Geometry: final body of the model. Coordinates: model frame, mm. A direction names the side the tool comes from. Give positions to 0.01 mm unless a question says otherwise; leave off trailing zeros. Write each loop counter-clockwise with the first axis right and the second up, starting at its lowest first coordinate (ties: lowest second). Pieces come first, ordered by that corner, then holes. Notation, with made-up numbers: (-6.5, 38.25) -> (27.5, 38.25) arc R28 ccw to (27.5, 65.25) -> close; hole circle Ø2 at (9.5, 31). An arc over 180 degrees is marked (long way). Answer in a Markdown table with one row per item. Add a question column.
Item 1: Material intervals for probe 1 along Z at (x, y) = (0, 4); probe 2 along Y at (x, z) = (12, -5.25); probe 3 along Z at (x, y) = (0, 48), sorted ascending. Write a range as from..to.
Item 2: Section query B-B on z = 0. Output: boundary loops of the cut face in (x, y), plus the area to 3 significant figures.
Item 3: Section query C-C on y = 80.5. Output: boundary loops of the cut face in (x, z), plus the area to 3 significant figures.
Item 4: Draft query along X for faces 4 (the cylindrical face through (14.07, 11.89, 4.43)), 5 (the flat face through (0, 77.8, 0)), 6 (the flat face through (-1, 12.9, -12)). Return one class per face: +X half, -X half, draft (parallel to the pull), parting line (faces both ways), or undercut.
Item 5: First-contact query: P1, Ø8, axis at x = -8.5, y = 20, coming from the +Z side; P2, Ø1.5, axis at y = 74.5, z = -6.5, coming from the +X side; P3, Ø8, axis at x = 7, y = 16.5, coming from the -Z side. Flat tips, straight axial feed; report the tip coordinate or a pass-through.
Item 6: Section query A-A on x = 0. Output: boundary loops of the cut face in (y, z).
Item 7: Section query D-D on y = 58. Output: boundary loops of the cut face in (x, z), plus the area to 3 significant figures.
Item 8: Access query for faces 1 (the cylindrical face through (11.207, 43.466, 3.529)), 2 (the flat face through (0, 10, 0)), 3 (the cylindrical face through (0, 83, -2)). Directions: +Z, -Z, +X, -X, +Y, -Y. A direction counts if a zero-diameter tool reaches every point of the face in a straight line with its end or side. Return the directions, or none.
Autodesk Fusion 360 part; units mm, degrees
sketch "Sketch1" plane through (0, 0, 0) normal (0, 1, 0) x (1, 0, 0)
  circle A0 centre (0, 0) radius 11.75
  dimension "d1" = 23.5
extrude "Extrude1" add sketch "Sketch1" along normal blind 87.8
sketch "Sketch2" plane through (0, 0, 0) normal (0, -1, 0) x (1, 0, 0)
  circle A0 centre (0, 0) radius 11.75
  circle A1 centre (0, 0) radius 2
  dimension "d4" = 4
extrude "Extrude2" cut sketch "Sketch2" against normal blind 10 contours A1
sketch "Sketch3" plane through (0, 87.8, 0) normal (0, 1, 0) x (-1, 0, 0)
  circle A0 centre (0, 0) radius 11.75
  circle A1 centre (0, 0) radius 2
  dimension "d7" = 4
extrude "Extrude3" cut sketch "Sketch3" against normal blind 10 contours A1
sketch "Sketch4" plane through (0, 0, 0) normal (0, -1, 0) x (1, 0, 0)
  circle A0 centre (0, 0) radius 2
  circle A1 centre (0, 0) radius 11.75
  circle A2 centre (0, 0) radius 14.75
  dimension "d10" = 3
extrude "Extrude4" add sketch "Sketch4" against normal blind 2 from surface at -10.9 contours A2
extrude "Extrude5" add sketch "Sketch4" along normal blind 2 from surface at -76.9 contours A2
Findings below:
| question | item | result |
|---|---|---|
| 1 | probe 1 | z = -11.75..-2, 2..11.75 |
| 1 | probe 2 | y = 10.9..12.9, 74.9..76.9 |
| 1 | probe 3 | z = -11.75..11.75 |
| 2 | outline | (-14.75, 10.9) -> (-11.75, 10.9) -> (-11.75, 0) -> (-2, 0) -> (-2, 10) -> (2, 10) -> (2, 0) -> (11.75, 0) -> (11.75, 10.9) -> (14.75, 10.9) -> (14.75, 12.9) -> (11.75, 12.9) -> (11.75, 74.9) -> (14.75, 74.9) -> (14.75, 76.9) -> (11.75, 76.9) -> (11.75, 87.8) -> (2, 87.8) -> (2, 77.8) -> (-2, 77.8) -> (-2, 87.8) -> (-11.75, 87.8) -> (-11.75, 76.9) -> (-14.75, 76.9) -> (-14.75, 74.9) -> (-11.75, 74.9) -> (-11.75, 12.9) -> (-14.75, 12.9) -> close |
| 2 | area | 2,010 mm^2 |
| 3 | outline | circle Ø23.5 at (0, 0); hole circle Ø4 at (0, 0) |
| 3 | area | 421 mm^2 |
| 4 | face 4 | parting line |
| 4 | face 5 | undercut |
| 4 | face 6 | draft |
| 5 | P1 | stops at z = 10.85 |
| 5 | P2 | stops at x = 13.53 |
| 5 | P3 | stops at z = -13.78 |
| 6 | outline | (0, -11.75) -> (10.9, -11.75) -> (10.9, -14.75) -> (12.9, -14.75) -> (12.9, -11.75) -> (74.9, -11.75) -> (74.9, -14.75) -> (76.9, -14.75) -> (76.9, -11.75) -> (87.8, -11.75) -> (87.8, -2) -> (77.8, -2) -> (77.8, 2) -> (87.8, 2) -> (87.8, 11.75) -> (76.9, 11.75) -> (76.9, 14.75) -> (74.9, 14.75) -> (74.9, 11.75) -> (12.9, 11.75) -> (12.9, 14.75) -> (10.9, 14.75) -> (10.9, 11.75) -> (0, 11.75) -> (0, 2) -> (10, 2) -> (10, -2) -> (0, -2) -> close |
| 7 | outline | circle Ø23.5 at (0, 0) |
| 7 | area | 434 mm^2 |
| 8 | face 1 | none |
| 8 | face 2 | -Y |
| 8 | face 3 | +Y |
